Autodesk Inventor part; units mm, degrees
ref_plane "YZ Plane" through (0, 0, 0) normal (1, 0, 0) x (0, 1, 0)
ref_plane "XZ Plane" through (0, 0, 0) normal (0, 1, 0) x (-1, 0, 0)
ref_plane "XY Plane" through (0, 0, 0) normal (0, 0, 1) x (1, 0, 0)
sketch "Sketch3" plane through (0, 0, 0) normal (0, 0, 1) x (1, 0, 0)
  line L0 (-163.0852, 54.3849) -> (-53.0852, 54.3849)
  line L1 (-53.0852, 54.3849) -> (-53.0852, -105.6151)
  line L2 (-53.0852, -105.6151) -> (-163.0852, -105.6151)
  line L3 (-163.0852, -105.6151) -> (-163.0852, 54.3849)
  point P0 (0, 0)
  dimension "d2" = 110
  dimension "d3" = 160
  dimension "d4" = 110
extrude "Extrusion1" add sketch "Sketch3" along normal blind 50
sketch "Sketch4" plane through (0, 0, 50) normal (0, 0, 1) x (1, 0, 0)
  point P0 (0, 0)
sketch "Sketch5" plane through (0, 0, 50) normal (0, 0, 1) x (1, 0, 0)
  line L0 (-163.0852, 54.3849) -> (-163.0852, -105.6151)
  line L1 (-163.0852, 54.3849) -> (-163.0852, 49.3849)
  line L2 (-163.0852, 49.3849) -> (-158.0852, 49.3849)
  line L3 (-158.0852, 49.3849) -> (-158.0852, -100.6151)
  line L4 (-158.0852, -100.6151) -> (-58.0852, -100.6151)
  line L5 (-58.0852, -100.6151) -> (-58.0852, 49.3849)
  line L6 (-58.0852, 49.3849) -> (-158.0852, 49.3849)
  point P0 (0, 0)
  dimension "d7" = 5
  dimension "d8" = 5
  dimension "d9" = 150
  dimension "d10" = 100
extrude "Extrusion2" cut sketch "Sketch5" against normal blind 45
sketch "Sketch6" plane through (-163.0852, 54.3849, 0) normal (0, 1, 0) x (1, 0, 0)
  line L0 (5, -5) -> (105, -5)
  line L1 (100.1792, -33.0786) -> (6.8805, -33.0786)
  line L2 (6.8805, -33.0786) -> (6.8805, -5)
  line L3 (6.8805, -5) -> (100.1792, -5)
  line L4 (100.1792, -5) -> (100.1792, -33.0786)
  point P0 (163.0852, 0)
extrude "Extrusion3" cut sketch "Sketch6" against normal blind 45
sketch "Sketch7" plane through (-163.0852, -105.6151, 0) normal (-1, 0, 0) x (0, 0, 1)
  line L0 (29.4052, 149.2988) -> (11.027, 149.2988)
  line L1 (11.027, 149.2988) -> (11.027, 85.399)
  line L2 (11.027, 85.399) -> (29.4052, 85.399)
  line L3 (29.4052, 85.399) -> (29.4052, 149.2988)
  line L4 (24.0331, 12.7342) -> (13.2889, 12.7342)
  line L5 (13.2889, 12.7342) -> (13.2889, 30.8297)
  line L6 (13.2889, 30.8297) -> (24.0331, 30.8297)
  line L7 (24.0331, 30.8297) -> (24.0331, 12.7342)
  point P0 (0, 105.6151)
extrude "Extrusion4" cut sketch "Sketch7" against normal blind 45 contours L3 L2 L1 L0
extrude "Extrusion5" cut sketch "Sketch7" against normal blind 45 contours L4 L5 L6 L7
sketch "Sketch8" plane through (-58.0852, -100.6151, 50) normal (-1, 0, 0) x (0, 0, 1)
  line L0 (-38.973, 144.2988) -> (-38.973, 80.399)
  line L1 (-9.5905, 135.2241) -> (-38.973, 135.2241)
  line L2 (-38.973, 135.2241) -> (-38.973, 98.4676)
  line L3 (-38.973, 98.4676) -> (-9.5905, 98.4676)
  line L4 (-9.5905, 98.4676) -> (-9.5905, 135.2241)
  point P0 (-50, 100.6151)
extrude "Extrusion6" cut sketch "Sketch8" against normal blind 45
properties material "Rubber"
Can you work these out from the model? Positions are in its coordinate system, mm. A direction names the side the tool comes from. Coordinates: 2 decimals unless noted, no trailing zeros. Write each loop counter-clockwise with the first axis right and the second up, starting at its lowest first coordinate (ties: lowest second). Pieces come first, ordered by that corner, then holes.
Q1. For P1, Ø6, axis at x = -101.5, z = 21.5, coming from the +Y side; P2, Ø4, axis at y = -77.5, z = 20, coming from the -X side; P3, Ø12, axis at y = 19.5, z = 26, coming from the +X side, each with a flat end and sliding along its axis, tell me the tip position at first contact or that it passes through.
Results found:
P1: stops at y = -100.62
P2: stops at x = -58.09
P3: stops at x = -158.09
Q2. Please list where these lines run through material, in increasing order: L1, parallel to Y at x = -118, z = 37.5; L2, parallel to X at y = -47.5, z = 44.5; L3, parallel to Z at x = -68, y = 16.
Results found:
L1: y = -105.62 to -100.62, 49.38 to 54.38
L2: x = -163.09 to -158.09, -58.09 to -53.09
L3: z = 0 to 5
Q3. Imagine slicing it at D-D, the plane y = -90. List the corners of the cut face in (x, z) for me.
Results found:
outline: (-163.09, 0) - (-53.09, 0) - (-53.09, 50) - (-58.09, 50) - (-58.09, 5) - (-158.09, 5) - (-158.09, 13.29) - (-163.09, 13.29) - close; (-163.09, 24.03) - (-158.09, 24.03) - (-158.09, 50) - (-163.09, 50) - close
Q4. Imagine slicing it at A-A, the plane y = 15. List the corners of the cut face in (x, z) for me, plus the area to 3 significant figures.
Results found:
outline: (-163.09, 0) - (-53.09, 0) - (-53.09, 11.03) - (-58.09, 11.03) - (-58.09, 5) - (-158.09, 5) - (-158.09, 11.03) - (-163.09, 11.03) - close; (-163.09, 29.41) - (-158.09, 29.41) - (-158.09, 50) - (-163.09, 50) - close; (-58.09, 40.41) - (-53.09, 40.41) - (-53.09, 50) - (-58.09, 50) - close
area: 761 mm2
Q5. Imagine slicing it at B-B, the plane z = 20. List the corners of the cut face in (x, y) for me.
Results found:
outline: (-163.09, -105.62) - (-53.09, -105.62) - (-53.09, -2.15) - (-58.09, -2.15) - (-58.09, -100.62) - (-158.09, -100.62) - (-158.09, -92.88) - (-163.09, -92.88) - close; (-163.09, -74.79) - (-158.09, -74.79) - (-158.09, -20.22) - (-163.09, -20.22) - close; (-163.09, 43.68) - (-158.09, 43.68) - (-158.09, 49.38) - (-156.2, 49.38) - (-156.2, 54.38) - (-163.09, 54.38) - close; (-62.91, 49.38) - (-58.09, 49.38) - (-58.09, 34.61) - (-53.09, 34.61) - (-53.09, 54.38) - (-62.91, 54.38) - close
Q6. Which directions (+Z, -Z, +X, -X, +Y, -Y) give clear straight access to the entire face, cutting with the end or side of a thin tool? Please do faces 5 (the face through (-62.906, 52, 19)), 6 (the face through (-56, 16, 40.41)), 7 (the face through (-161, 12, 11.027)), 8 (the face through (-158.085, -41, 28)), 9 (the face through (-56, 16, 11.027)).
Results found:
face 5: +Y
face 6: +X
face 7: -X
face 8: +Z
face 9: +X, -X
Q7. Imagine slicing it at C-C, the plane x = -111.5. List the corners of the cut face in (y, z) for me.
Results found:
outline: (-105.62, 0) - (54.38, 0) - (54.38, 5) - (-100.62, 5) - (-100.62, 50) - (-105.62, 50) - close; (49.38, 33.08) - (54.38, 33.08) - (54.38, 50) - (49.38, 50) - close
Q8. If we mould it in two halves opening along Z, with no side actions, what happens to faces 1 (the face through (-161, -25, 50)), 2 (the face through (-161, -20.216, 20)), 3 (the face through (-109, -24, 0)), 4 (the face through (-161, -84, 24.033))? For each: +Z half, -Z half, draft (parallel to the pull), parting line (faces both ways), or undercut.
Results found:
face 1: +Z half
face 2: undercut
face 3: -Z half
face 4: undercut
